from build123d import *

# Parameters (mm, degrees)
MOVE_BODY_2_DEPTH    = 3000
SKETCH_6_OUTSIDE_W   = 652.406
SKETCH_6_OUTSIDE_H   = 3602.406
SKETCH_6_OUTSIDE_W_2 = 50
SKETCH_6_OUTSIDE_H_2 = 799.25
CUT_EXTRUDE_1_DEPTH  = 3003.033019472


# Read off the part's stored shape, not the designer's step: Тело-Переместить/Копировать2
with BuildPart() as part:
    # Move Body 2 outline → Move Body 2 (new body)
    with BuildSketch(Plane(origin=(0, 0, 0), x_dir=(1, 0, 0), z_dir=(0, 1, 0))):
        with BuildLine():
            Line((-50, 47.75), (-50, 46.25))
            Line((-50, 46.25), (-49.25, 46.25))
            Line((-49.25, 46.25), (-49.25, 47.75))
            ThreePointArc((-49.25, 47.75), (-49.030330086, 48.280330086), (-48.5, 48.5))
            Line((-48.5, 48.5), (-1.5, 48.5))
            ThreePointArc((-1.5, 48.5), (-0.969669914, 48.280330086), (-0.75, 47.75))
            Line((-0.75, 47.75), (-0.75, -47.75))
            ThreePointArc((-0.75, -47.75), (-0.969669914, -48.280330086), (-1.5, -48.5))
            Line((-1.5, -48.5), (-48.5, -48.5))
            ThreePointArc((-48.5, -48.5), (-49.030330086, -48.280330086), (-49.25, -47.75))
            Line((-49.25, -47.75), (-49.25, -46.25))
            Line((-49.25, -46.25), (-50, -46.25))
            Line((-50, -46.25), (-50, -47.75))
            ThreePointArc((-50, -47.75), (-49.560660172, -48.810660172), (-48.5, -49.25))
            Line((-48.5, -49.25), (-1.5, -49.25))
            ThreePointArc((-1.5, -49.25), (-0.439339828, -48.810660172), (0, -47.75))
            Line((0, -47.75), (0, 47.75))
            ThreePointArc((0, 47.75), (-0.439339828, 48.810660172), (-1.5, 49.25))
            Line((-1.5, 49.25), (-48.5, 49.25))
            ThreePointArc((-48.5, 49.25), (-49.560660172, 48.810660172), (-50, 47.75))
        make_face()
    extrude(amount=MOVE_BODY_2_DEPTH)

    # Эскиз6 outside → Вырез-Вытянуть1 (cut, through all)
    with BuildSketch(Plane.XY.offset(49.25)):
        with Locations((-25, 1500)):
            Rectangle(SKETCH_6_OUTSIDE_W, SKETCH_6_OUTSIDE_H)
        with Locations((-25, 2600.375)):
            Rectangle(SKETCH_6_OUTSIDE_W_2, SKETCH_6_OUTSIDE_H_2, mode=Mode.SUBTRACT)
    extrude(amount=-CUT_EXTRUDE_1_DEPTH, mode=Mode.SUBTRACT)


solid = part.part
Geometry: final body of the model. Coordinates: model frame, mm. Give positions to 0.01 mm unless a question says otherwise; leave off trailing zeros. Order: outer loops, then holes, each group sorted by start corner. A loop starts at its lowest first (then second) coordinate and runs counter-clockwise, first axis right, second up. Notation, with made-up numbers: (14.5, 59.5) -> (69.5, 59.5) arc R19 ccw to (69.5, 78.5) -> close; hole circle Ø10 at (57.25, 57). An arc over 180 degrees is marked (long way). Answer as a JSON object with one key per item and string values.
Q1. Material intervals for probe 1 along Z at (x, y) = (-46.5, 2732.5); probe 2 along X at (y, z) = (2569.5, 33), sorted ascending.
Entries:
{"probe 1": "z = -49.25 to -48.5, 48.5 to 49.25", "probe 2": "x = -0.75 to 0"}
Q2. First-contact query: pin 1 (0.8 mm diameter, centred on x = -49.5, y = 2406, fed in from +Z); pin 2 (0.6 mm diameter, centred on x = -49.5, y = 2762, fed in from -Z); pin 3 (4 mm diameter, centred on y = 2707, z = -15, fed in from -X). Flat tips, straight axial feed; report the tip coordinate or a pass-through.
Entries:
{"pin 1": "stops at z = 49.12", "pin 2": "stops at z = -49.08", "pin 3": "stops at x = -0.75"}
Q3. Section A-A (x = -29.5). Output: boundary loops of the cut face in (y, z), plus the area to 3 significant figures.
Entries:
{"outline": "(2200.75, -49.25) -> (3000, -49.25) -> (3000, -48.5) -> (2200.75, -48.5) -> close; (2200.75, 48.5) -> (3000, 48.5) -> (3000, 49.25) -> (2200.75, 49.25) -> close", "area": "1,200 mm^2"}
Q4. Section B-B (y = 2892). Output: boundary loops of the cut face in (x, z).
Entries:
{"outline": "(-50, -47.75) arc R1.5 ccw to (-48.5, -49.25) -> (-1.5, -49.25) arc R1.5 ccw to (0, -47.75) -> (0, 47.75) arc R1.5 ccw to (-1.5, 49.25) -> (-48.5, 49.25) arc R1.5 ccw to (-50, 47.75) -> (-50, 46.25) -> (-49.25, 46.25) -> (-49.25, 47.75) arc R0.75 cw to (-48.5, 48.5) -> (-1.5, 48.5) arc R0.75 cw to (-0.75, 47.75) -> (-0.75, -47.75) arc R0.75 cw to (-1.5, -48.5) -> (-48.5, -48.5) arc R0.75 cw to (-49.25, -47.75) -> (-49.25, -46.25) -> (-50, -46.25) -> close"}
Q5. Draft query along Z for faces 1 (the flat face through (0, 2595, 1)), 2 (the flat face through (-25, 2595, -49.25)), 3 (the flat face through (-0.75, 2595, -1)), 4 (the flat face through (-25, 2595, 49.25)). Return one class per face: released by +Z, released by -Z, zero draft, split by the parting line, or undercut.
Entries:
{"face 1": "zero draft", "face 2": "released by -Z", "face 3": "undercut", "face 4": "released by +Z"}
Q6. Section C-C (z = 1.5). Output: boundary loops of the cut face in (x, y), plus the area to 3 significant figures.
Entries:
{"outline": "(-0.75, 2200.75) -> (0, 2200.75) -> (0, 3000) -> (-0.75, 3000) -> close", "area": "599 mm^2"}
